Geometry check sheet. Reference: drawing and pictorial views, mm from the part's lowest x, y, z. A direction names the side the tool comes from. Round coordinates to 2 decimals unless told otherwise and drop trailing zeros. Order: outer loops, then holes, each group sorted by start corner. A loop starts at its lowest first (then second) coordinate and runs counter-clockwise, first axis right, second up.
(1) Set-up check for the marked faces 4 and 5: record each of +Z, -Z, +X, -X, +Y, -Y from which the full face is reachable in a straight line by a thin tool's end or side.
(2) Go/stop test with a flat-tipped pin: pin 1 (4 mm diameter, centred on y = 23.5, z = 14.5, fed in from -X). Record where the tip stops, or that it passes through.
(3) Sectioned sample at A-A (x = 16). Record the boundary of the cut face in (y, z), plus the area to 3 significant figures.
(4) Sectioned sample at C-C (y = 26). Record the boundary of the cut face in (x, z), plus the area to 3 significant figures.
(5) Release check for a two-part mould opening along Y. For the marked faces 1, 2 and 3 record: +Y half, -Y half, draft (parallel to the pull), parting line (faces both ways), or undercut.
(6) Material ranges on line 1 along Y through (x, z) = (15, 18); line 2 along X through (y, z) = (36.5, 32.5), recorded low to high.
(7) Sectioned sample at B-B (z = 34). Record the boundary of the cut face in (x, y).
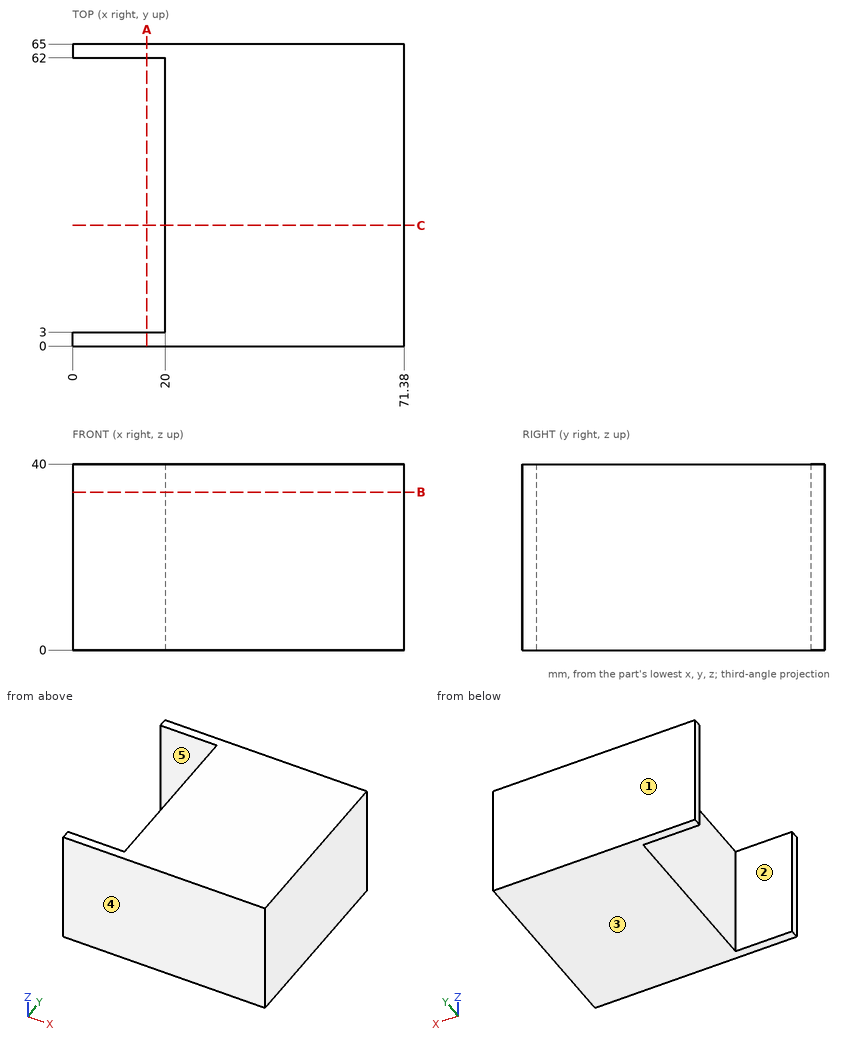
Answer below:
1. face 4: +Z, -Z, +X, -X, -Y
1. face 5: +Z, -Z, -X
2. pin 1: stops at x = 20
3. outline: (0, 0) - (3, 0) - (3, 40) - (0, 40) - close; (62, 0) - (65, 0) - (65, 40) - (62, 40) - close
3. area: 240 mm2
4. outline: (20, 0) - (71.38, 0) - (71.38, 40) - (20, 40) - close
4. area: 2,060 mm2
5. face 1: +Y half
5. face 2: undercut
5. face 3: draft
6. line 1: y = 0 to 3, 62 to 65
6. line 2: x = 20 to 71.38
7. outline: (0, 0) - (71.38, 0) - (71.38, 65) - (0, 65) - (0, 62) - (20, 62) - (20, 3) - (0, 3) - close
